Verification items for the finished model (mm, model axes). Face numbers are marked on the shaded views. A direction names the side the tool comes from. Coordinates: 2 decimals unless noted, no trailing zeros. Order: outer loops, then holes, each group sorted by start corner. A loop starts at its lowest first (then second) coordinate and runs counter-clockwise, first axis right, second up. Notation, with made-up numbers: M 7.5,-22 L 49.5,-22 A29 cw 49.5,-1 Z; hole C 10,59 d8. An arc over 180 degrees is marked long. Return JSON: item names as keys, results as strings. Group by question number.
Q1. Section check C-C, the plane x = 0. Enter the section's corners in (y, z), then the cut area to 3 significant figures.
Q2. Thickness scan on probe 1 along X at (y, z) = (0, -34.1); probe 2 along Z at (x, y) = (10, -11.25); probe 3 along Z at (x, y) = (-41, 9). Record the ranges inside material, lowest first.
Q3. Section check A-A, the plane y = 0. Count the separate pieces of the cut face and the enclosed holes in it, then the cut area to 3 significant figures.
Q4. Access from +Z, -Z, +X, -X, +Y, -Y to the whole of each face (thin tool, end or side, straight path). Record for the marked faces 5 and 6.
Q5. Go/stop test with flat-tipped pins: pin 1 Ø4 at (y, z) = (-3.5, -70) entering from -X; pin 2 Ø4.5 at (x, z) = (7, -33.5) entering from +Y; pin 3 Ø1.5 at (y, z) = (-7.5, -101.5) entering from +X. Record where each tip stops, or that it passes through.
Q6. Mould release check, pull along X, two halves, no side actions. Record for the marked faces 1, 2, 3 and 4: pulls with the +X half, pulls with the -X half, needs draft (parallel to the pull), parting line crosses it, or undercut.
Q7. Section check B-B, the plane z = -107.5. Enter the section's corners in (x, y), then the cut area to 3 significant figures.
Q8. Section check D-D, the plane x = 12. Enter the section's corners in (y, z), then the cut area to 4 significant figures.
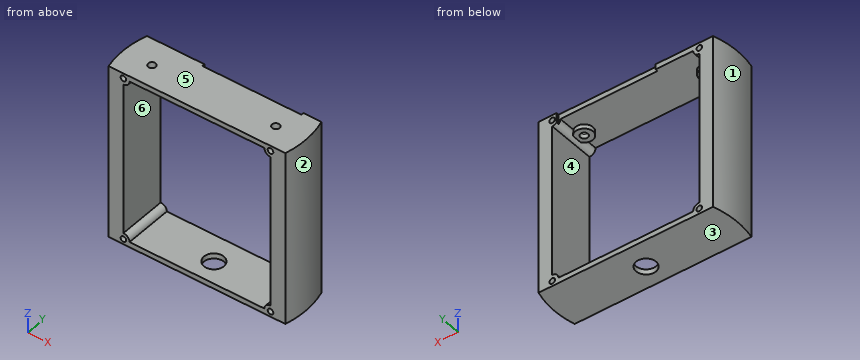
from build123d import *

# Parameters (mm, degrees)
PAD005_DEPTH    = 100
SKETCH007_R     = 1.6
POCKET001_DEPTH = 27.501
SKETCH008_R     = 2.15
POCKET002_DEPTH = 50
SKETCH014_R     = 5
SKETCH014_R_2   = 2.15
PAD010_DEPTH    = 2.5
SKETCH019_W     = 56.540354
SKETCH019_H     = 5.490008
POCKET_DEPTH    = 1.5
SKETCH020_R     = 5.7
POCKET004_DEPTH = 10


with BuildPart() as part:
    # Sketch006 → Pad005 (new body)
    with BuildSketch(Plane.XY):
        with BuildLine():
            Line((-49.789557, 15), (49.789557, 15))
            ThreePointArc((50.475241, -12.5), (51.983843, 1.296164), (49.789557, 15))
            Line((-50.475241, -12.5), (50.475241, -12.5))
            ThreePointArc((-49.789557, 15), (-51.983843, 1.296164), (-50.475241, -12.5))
        make_face()
    extrude(amount=PAD005_DEPTH)

    # Sketch007 (on Face3 of Pad005) → Pocket001 (cut, through all)
    with BuildSketch(Plane.XZ.offset(12.5)):
        with Locations((-42, 97)):
            Circle(SKETCH007_R)
        with Locations((42, 97)):
            Circle(SKETCH007_R)
        with Locations((42, 3)):
            Circle(SKETCH007_R)
        with Locations((-42, 3)):
            Circle(SKETCH007_R)
        with BuildLine():
            ThreePointArc((-42, 93.5), (-39.525126, 94.525126), (-38.5, 97))
            Line((-38.5, 97), (38.5, 97))
            ThreePointArc((38.5, 97), (39.525126, 94.525126), (42, 93.5))
            Line((42, 93.5), (42, 6.5))
            ThreePointArc((42, 6.5), (39.525126, 5.474874), (38.5, 3))
            Line((38.5, 3), (-38.5, 3))
            ThreePointArc((-38.5, 3), (-39.525126, 5.474874), (-42, 6.5))
            Line((-42, 6.5), (-42, 93.5))
        make_face()
    extrude(amount=-POCKET001_DEPTH, mode=Mode.SUBTRACT)

    # Sketch008 (on Face4 of Pocket001) → Pocket002 (cut)
    with BuildSketch(Plane.XY.offset(100)):
        with Locations((-35.355339, 0)):
            Circle(SKETCH008_R)
        with Locations((35.355339, 0)):
            Circle(SKETCH008_R)
    extrude(amount=-POCKET002_DEPTH, mode=Mode.SUBTRACT)

    # Sketch014 (on Face10 of Pocket002) → Pad010 (join)
    with BuildSketch(Plane(origin=(0, 0, 97), x_dir=(1, 0, 0), z_dir=(0, 0, -1))):
        with Locations((-35.355339, 0)):
            Circle(SKETCH014_R)
        with Locations((-35.355339, 0)):
            Circle(SKETCH014_R_2, mode=Mode.SUBTRACT)
        with Locations((35.355339, 0)):
            Circle(SKETCH014_R)
        with Locations((35.355339, 0)):
            Circle(SKETCH014_R_2, mode=Mode.SUBTRACT)
    extrude(amount=PAD010_DEPTH)

    # Sketch019 (on Face1 of Pad010) → Pocket (cut)
    with BuildSketch(Plane(origin=(0, 15, 0), x_dir=(-1, 0, 0), z_dir=(0, 1, 0))):
        with Locations((-11.270177, 97.254996)):
            Rectangle(SKETCH019_W, SKETCH019_H)
    extrude(amount=-POCKET_DEPTH, mode=Mode.SUBTRACT)

    # Sketch020 (on Face2 of Pocket) → Pocket004 (cut)
    with BuildSketch(Plane(origin=(0, 0, 0), x_dir=(1, 0, 0), z_dir=(0, 0, -1))):
        Circle(SKETCH020_R)
    extrude(amount=-POCKET004_DEPTH, mode=Mode.SUBTRACT)


with BuildPart() as part_1:
    # Body006 placement: moved
    add(part.part.moved(Location((0, 0, -130.2))))


solid = part_1.part
Numbers:
{
 "1": {"outline": "M -12.5,-130.2 L -5.7,-130.2 L -5.7,-127.2 L -12.5,-127.2 Z; M -12.5,-33.2 L 13.5,-33.2 L 13.5,-30.2 L -12.5,-30.2 Z; M 5.7,-130.2 L 15,-130.2 L 15,-127.2 L 5.7,-127.2 Z", "area": "126 mm2"},
 "2": {"probe 1": "x = -52 to -43.32, -40.68 to -37.51, -33.21 to -30.36, 30.36 to 33.21, 37.51 to 40.68, 43.32 to 52", "probe 2": "z = -130.2 to -127.2, -33.2 to -30.2", "probe 3": "z = -130.2 to -128.45, -125.95 to -123.85, -36.55 to -34.45, -31.95 to -30.2"},
 "3": {"separate pieces": "3", "enclosed holes": "4", "area": "2,470 mm2"},
 "4": {"face 5": "+Z, +X, -X, +Y, -Y", "face 6": "+Y, -Y"},
 "5": {"pin 1": "stops at x = -51.98", "pin 2": "stops at y = 13.5", "pin 3": "stops at x = 51.56"},
 "6": {"face 1": "pulls with the -X half", "face 2": "pulls with the +X half", "face 3": "needs draft", "face 4": "undercut"},
 "7": {"outline": "M -50.48,-12.5 L -42,-12.5 L -42,15 L -49.79,15 A52 ccw Z; M 42,-12.5 L 50.48,-12.5 A52 ccw 49.79,15 L 42,15 Z", "area": "515 mm2"},
 "8": {"outline": "M -12.5,-130.2 L 15,-130.2 L 15,-127.2 L -12.5,-127.2 Z; M -12.5,-33.2 L 13.5,-33.2 L 13.5,-30.2 L -12.5,-30.2 Z", "area": "160.5 mm2"}
}
